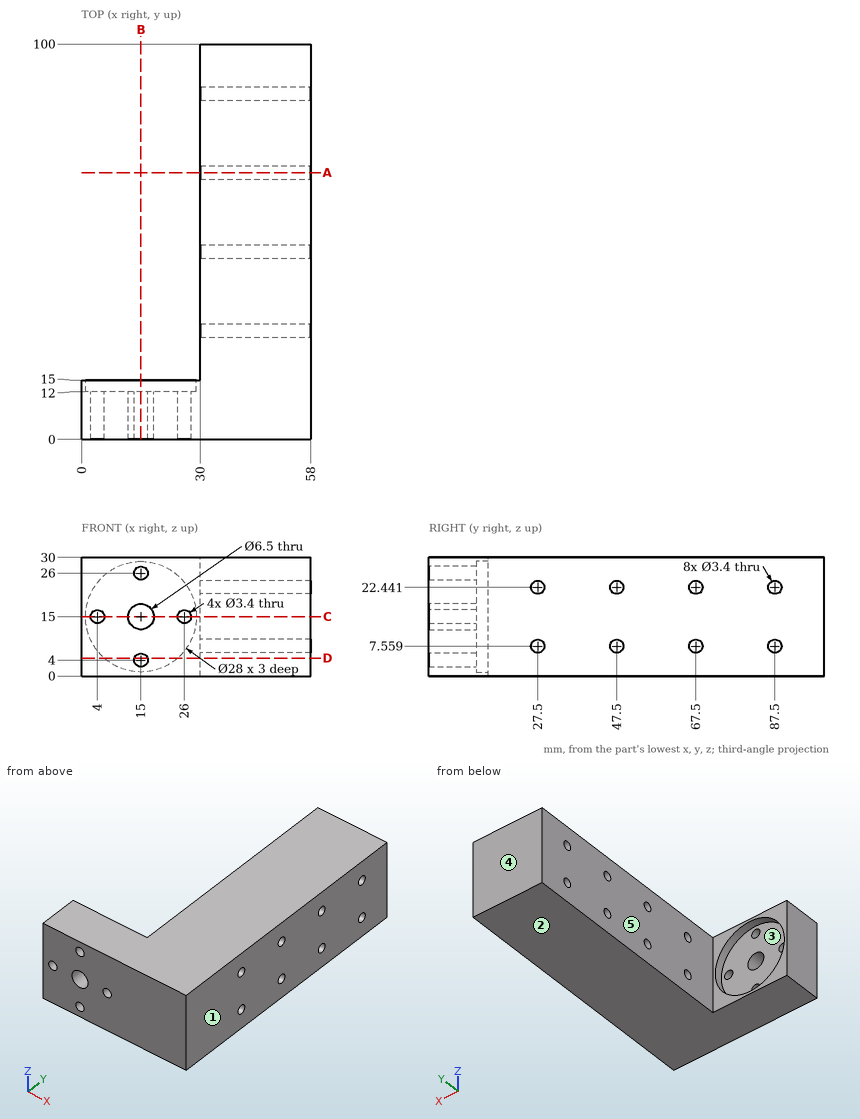
Source: three-view drawing plus pictorial views. Frame: mm from the lowest corner of the part. A direction names the side the tool comes from. Give positions to 0.01 mm unless a question says otherwise; leave off trailing zeros. Loops run counter-clockwise (first coordinate to the right, second up) from the corner with the lowest first, then second, coordinate; pieces in that order, holes last. Notation, with made-up numbers: (-39.5, -33) -> (-4.5, -33) arc R31 cw to (-4.5, -7) -> close; hole circle Ø7 at (-33, 44). An arc over 180 degrees is marked (long way). Use a Markdown table: item, result. Add a question column.
(1) First-contact query: pin 1 Ø4.5 at (y, z) = (87.5, 7.56) entering from -X; pin 2 Ø5.5 at (x, z) = (4, 15) entering from -Y; pin 3 Ø14 at (x, z) = (8, 13.5) entering from +Y; pin 4 Ø9 at (x, z) = (11.5, 20.5) entering from +Y. Flat tips, straight axial feed; report the tip coordinate or a pass-through.
(2) Section query C-C (z = 15). Output: boundary loops of the cut face in (x, y), then the cut area to 3 significant figures.
(3) Access query for the marked faces 4 and 5. Directions: +Z, -Z, +X, -X, +Y, -Y. A direction counts if a zero-diameter tool reaches every point of the face in a straight line with its end or side. Return the directions, or none.
(4) Section query A-A (y = 67.5). Output: boundary loops of the cut face in (x, z), then the cut area to 3 significant figures.
(5) Section query B-B (x = 15). Output: boundary loops of the cut face in (y, z).
(6) Ray query, line 1 (Z direction, x = 43, y = 27.5); line 2 (X direction, y = 7.25, z = 15); line 3 (Y direction, x = 38, z = 7.5). Return the intervals inside material, ascending.
(7) Section query D-D (z = 4.5). Output: boundary loops of the cut face in (x, y) (3 decimals).
(8) Pull-direction query (Z, two-part tool) for the marked faces 1, 2 and 3; classes: +Z half, -Z half, draft (parallel to the pull), parting line (faces both ways), or undercut.
Checked values:
| question | item | result |
|---|---|---|
| 1 | pin 1 | x = 30 |
| 1 | pin 2 | y = 0 |
| 1 | pin 3 | y = 15 |
| 1 | pin 4 | y = 12 |
| 2 | outline | (0, 0) -> (2.3, 0) -> (2.3, 12) -> (1, 12) -> (1, 15) -> (0, 15) -> close; (5.7, 0) -> (11.75, 0) -> (11.75, 12) -> (5.7, 12) -> close; (18.25, 0) -> (24.3, 0) -> (24.3, 12) -> (18.25, 12) -> close; (27.7, 0) -> (58, 0) -> (58, 100) -> (30, 100) -> (30, 15) -> (29, 15) -> (29, 12) -> (27.7, 12) -> close |
| 2 | area | 3,010 mm^2 |
| 3 | face 4 | +Z, -Z, +X, -X, +Y |
| 3 | face 5 | +Z, -Z, -X, +Y |
| 4 | outline | (30, 0) -> (58, 0) -> (58, 5.86) -> (30, 5.86) -> close; (30, 9.26) -> (58, 9.26) -> (58, 20.74) -> (30, 20.74) -> close; (30, 24.14) -> (58, 24.14) -> (58, 30) -> (30, 30) -> close |
| 4 | area | 650 mm^2 |
| 5 | outline | (0, 0) -> (15, 0) -> (15, 1) -> (12, 1) -> (12, 2.3) -> (0, 2.3) -> close; (0, 5.7) -> (12, 5.7) -> (12, 11.75) -> (0, 11.75) -> close; (0, 18.25) -> (12, 18.25) -> (12, 24.3) -> (0, 24.3) -> close; (0, 27.7) -> (12, 27.7) -> (12, 29) -> (15, 29) -> (15, 30) -> (0, 30) -> close |
| 6 | line 1 | 0 to 5.86, 9.26 to 20.74, 24.14 to 30 |
| 6 | line 2 | 0 to 2.3, 5.7 to 11.75, 18.25 to 24.3, 27.7 to 58 |
| 6 | line 3 | 0 to 25.8, 29.2 to 45.8, 49.2 to 65.8, 69.2 to 85.8, 89.2 to 100 |
| 7 | outline | (0, 0) -> (13.375, 0) -> (13.375, 12) -> (5.74, 12) -> (5.74, 15) -> (0, 15) -> close; (16.625, 0) -> (58, 0) -> (58, 100) -> (30, 100) -> (30, 15) -> (24.26, 15) -> (24.26, 12) -> (16.625, 12) -> close |
| 8 | face 1 | draft |
| 8 | face 2 | -Z half |
| 8 | face 3 | undercut |
